Geometry: final body of the model. Coordinates: model frame, mm. Coordinates: 2 decimals unless noted, no trailing zeros. Order: outer loops, then holes, each group sorted by start corner. A loop starts at its lowest first (then second) coordinate and runs counter-clockwise, first axis right, second up. Notation, with made-up numbers: (69.25, 76) -> (116.25, 76) arc R29 ccw to (116.25, 114) -> close; hole circle Ø9 at (76.5, 68.5). An arc over 180 degrees is marked (long way). Use one line per item in the form item = value.
```python
from build123d import *

# Parameters (mm, degrees)
BOSS_EXTRUDE1_DEPTH = 3
SKETCH2_W           = 15.500819923
SKETCH2_H           = 6.5
CUT_EXTRUDE1_DEPTH  = 176.817329233
SKETCH3_W           = 23
SKETCH3_H           = 12
CUT_EXTRUDE2_DEPTH  = 176.817329233
SKETCH4_W           = 6
SKETCH4_H           = 12
BOSS_EXTRUDE2_DEPTH = 4


with BuildPart() as part:
    # Sketch1 → Boss-Extrude1 (new body)
    with BuildSketch(Plane(origin=(0, 0, 0), x_dir=(1, 0, 0), z_dir=(0, 1, 0))):
        with BuildLine():
            Line((0, -91), (0, 91))
            Line((0, 91), (150.405230157, 26.996958875))
            ThreePointArc((150.405230157, 26.996958875), (123.000159405, 0.092778483), (150.219685616, -26.999106249))
            Line((150.219685616, -26.999106249), (0, -91))
        make_face()
    extrude(amount=BOSS_EXTRUDE1_DEPTH)

    # Sketch2 → Cut-Extrude1 (cut, through all)
    with BuildSketch(Plane(origin=(0, 3, 0), x_dir=(1, 0, 0), z_dir=(0, 1, 0))):
        with Locations((73.073381573, -42.257557828)):
            Rectangle(SKETCH2_W, SKETCH2_H)
    extrude(amount=-CUT_EXTRUDE1_DEPTH, mode=Mode.SUBTRACT)

    # Sketch3 → Cut-Extrude2 (cut, through all)
    with BuildSketch(Plane(origin=(0, 3, 0), x_dir=(1, 0, 0), z_dir=(0, 1, 0))):
        with Locations((82.780547291, 0)):
            Rectangle(SKETCH3_W, SKETCH3_H)
    extrude(amount=-CUT_EXTRUDE2_DEPTH, mode=Mode.SUBTRACT)

    # Sketch4 → Boss-Extrude2 (add)
    with BuildSketch(Plane(origin=(0, 3, 0), x_dir=(1, 0, 0), z_dir=(0, 1, 0))):
        with Locations((97.280547291, 0)):
            Rectangle(SKETCH4_W, SKETCH4_H)
        with Locations((68.280547291, 0)):
            Rectangle(SKETCH4_W, SKETCH4_H)
    extrude(amount=BOSS_EXTRUDE2_DEPTH)


solid = part.part
```
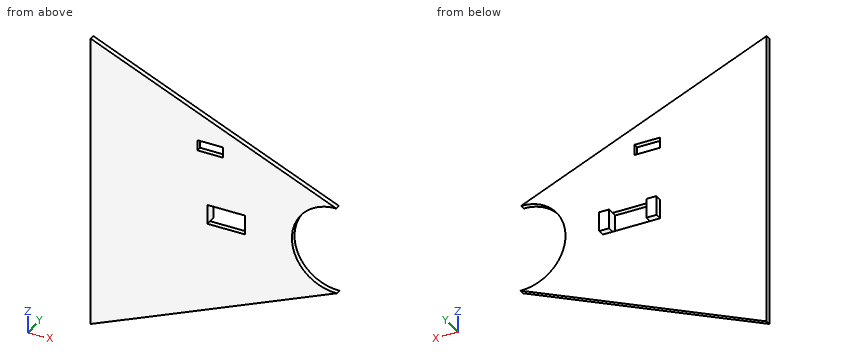
1) Section B-B, the plane y = 1.5. Output: boundary loops of the cut face in (x, z).
Results found:
outline = (0, -91) -> (150.41, -27) arc R27 cw (long way) to (150.22, 27) -> (0, 91) -> close; hole (65.32, 39.01) -> (80.82, 39.01) -> (80.82, 45.51) -> (65.32, 45.51) -> close; hole (71.28, -6) -> (94.28, -6) -> (94.28, 6) -> (71.28, 6) -> close
2) Contact query for flat-ended pins moving along their axis: P1, Ø1.5, axis at x = 76, y = 1, coming from the +Z side; P2, Ø8, axis at x = 82, z = -10, coming from the +Y side; P3, Ø1.2, axis at x = 67, y = 6, coming from the +Z side. Output: stop coordinate, or through.
Results found:
P1 = 58.94
P2 = 3
P3 = 6
3) Section C-C, the plane x = 130. Output: boundary loops of the cut face in (y, z).
Results found:
outline = (0, -35.68) -> (3, -35.68) -> (3, -18.14) -> (0, -18.14) -> close; (0, 18.14) -> (3, 18.14) -> (3, 35.61) -> (0, 35.61) -> close
4) Section A-A, the plane z = 0. Output: boundary loops of the cut face in (x, y), and give its area (3 significant figures).
Results found:
outline = (0, 0) -> (71.28, 0) -> (71.28, 7) -> (65.28, 7) -> (65.28, 3) -> (0, 3) -> close; (94.28, 0) -> (123, 0) -> (123, 3) -> (100.28, 3) -> (100.28, 7) -> (94.28, 7) -> close
area = 348 mm2
5) Material intervals for probe 1 along X at (y, z) = (4.75, -3); probe 2 along Z at (x, y) = (80, 2.5); probe 3 along Y at (x, z) = (85, -22), sorted ascending. Write a range as from..to.
Results found:
probe_1 = 65.28..71.28, 94.28..100.28
probe_2 = -56.96..-6, 6..39.01, 45.51..56.92
probe_3 = 0..3
6) Section D-D, the plane x = 86. Output: boundary loops of the cut face in (y, z).
Results found:
outline = (0, -54.4) -> (3, -54.4) -> (3, -6) -> (0, -6) -> close; (0, 6) -> (3, 6) -> (3, 54.36) -> (0, 54.36) -> close
